```python
from build123d import *

# Parameters (mm, degrees)
F1_DEPTH = 9
F2_R     = 1.25
F3_DEPTH = 1
F4_R     = 0.625
F5_R     = 0.625
F6_DEPTH = 1


with BuildPart() as f1:
    # F0 (on Top) → F1 (new body)
    with BuildSketch(Plane.XY):
        with BuildLine():
            Line((-24.9881935865, -2), (-29.9881935865, -2))
            add(Edge.make_bspline(
                [(-29.9881935865, -2), (-30.1957792579, -1.9806863621), (-30.8858297438, -1.9886899929), (-30.9737131442, -1.9691203625), (-32.3240056363, -2.0563246792), (-32.4695344233, -2.4918309621)],
                knots=[0, 0, 0, 0, 0.3435850183, 0.5315375028, 0.9674384772, 0.9674384772, 0.9674384772, 0.9674384772], degree=3))
            Line((-32.4695344233, -2.4918309621), (-32.4881935865, -10.0656754612))
            ThreePointArc((-32.4881935865, -10.0656754612), (-31.3797872361, -10.9135774988), (-29.9881935865, -11.0183134402))
            Line((-29.9881935865, -11.0183134402), (-25.0104854877, -11.0483904604))
            ThreePointArc((-25.0104854877, -11.0483904604), (-23.5833955913, -10.9234349089), (-22.4881935865, -10))
            Line((-22.4881935865, -10), (-22.4881935865, -2.6204695865))
            ThreePointArc((-22.4881935865, -2.6204695865), (-23.6846353493, -2.0944376038), (-24.9881935865, -2))
        make_face()
        Polygon((-27.4881935865, 0), (-29.9881935865, 0), (-29.9881935865, -2), (-24.9881935865, -2), (-24.9881935865, 0), align=None)
        Polygon((-25.0104854877, -11.0483904604), (-29.9881935865, -11.0183134402), (-29.9881935865, -12), (-27.4881935865, -12), (-25.0128299031, -12), align=None)
    extrude(amount=F1_DEPTH)

    # F2 (on face) → F3 (join)
    with BuildSketch(Plane.XY.offset(9)):
        with Locations((-29.9974028021, -3.6542222369)):
            Circle(F2_R)
        with Locations((-24.9764043838, -3.7198562641)):
            Circle(F2_R)
        with BuildLine():
            Line((-24.4942996651, -8.7319174781), (-30.507825315, -8.6252950132))
            ThreePointArc((-30.507825315, -8.6252950132), (-27.5242896541, -9.9886223537), (-24.4942996651, -8.7319174781))
        make_face()
    extrude(amount=F3_DEPTH)

    # F4 (on face) + F5 (on face) → F6 (cut)
    with BuildSketch(Plane.XY.offset(10)):
        with Locations((-29.9974028021, -3.6542222369)):
            Circle(F4_R)
    with BuildSketch(Plane.XY.offset(10)):
        with Locations((-24.9764043838, -3.7198562641)):
            Circle(F5_R)
    extrude(amount=F6_DEPTH, mode=Mode.SUBTRACT)


solid = f1.part
```
CAD build for the part. Positions are in the model's coordinates, mm. A direction names the side the tool comes from. Round coordinates to 2 decimals unless told otherwise and drop trailing zeros. Order: outer loops, then holes, each group sorted by start corner. A loop starts at its lowest first (then second) coordinate and runs counter-clockwise, first axis right, second up.
Item 1: Tool access for faces 4 (the face through (-28, -6, 0)), 5 (the face through (-31.246, -3.599, 9.493)): list every direction of +Z, -Z, +X, -X, +Y, -Y with a clear straight run to the whole face (end or side of a thin tool).
Item 2: Saw through at B-B on y = -3. Write the cut outline in (x, z), then the cut area to 3 significant figures.
Item 3: Saw through at C-C on x = -28.5. Write the cut outline in (y, z).
Item 4: Saw through at A-A on x = -25.75. Write the cut outline in (y, z), then the cut area to 3 significant figures.
Item 5: Probe line 1 along Z through (x, y) = (-25.25, -8); line 2 along X through (y, z) = (-9, 6.5); line 3 along X through (y, z) = (-10.5, 7). List the from-to ranges inside material, lowest first.
Item 6: Mould opens along X. For faces 1 (the face through (-31.398, -10.906, 4.437)), 2 (the face through (-28, -9, 10)), 3 (the face through (-22.488, -6, 4)) say: pulls with the +X half, pulls with the -X half, needs draft (parallel to the pull), parting line crosses it, or undercut.
Item 7: Saw through at D-D on y = -8. Write the cut outline in (x, z), then the cut area to 3 significant figures.
Item 8: Pin check, flat tips, straight feed: pin 1 (3 mm diameter, centred on y = -2, z = 1, fed in from -X); pin 2 (1.6 mm diameter, centred on y = -1.5, z = 6.5, fed in from +X). Stop position of each tip, or through.
Reported:
1. face 4: -Z, +X, -X, +Y, -Y
1. face 5: +Z
2. outline: (-32.47, 0) - (-22.49, 0) - (-22.49, 9) - (-23.95, 9) - (-23.95, 10) - (-26, 10) - (-26, 9) - (-28.93, 9) - (-28.93, 10) - (-31.06, 10) - (-31.06, 9) - (-32.47, 9) - close
2. area: 94.0 mm2
3. outline: (-12, 0) - (0, 0) - (0, 9) - (-8.66, 9) - (-8.66, 10) - (-9.85, 10) - (-9.85, 9) - (-12, 9) - close
4. outline: (-12, 0) - (0, 0) - (0, 9) - (-2.74, 9) - (-2.74, 10) - (-4.7, 10) - (-4.7, 9) - (-8.71, 9) - (-8.71, 10) - (-9.62, 10) - (-9.62, 9) - (-12, 9) - close
4. area: 111 mm2
5. line 1: z = 0 to 9
5. line 2: x = -32.49 to -22.49
5. line 3: x = -32.08 to -22.91
6. face 1: undercut
6. face 2: needs draft
6. face 3: pulls with the +X half
7. outline: (-32.48, 0) - (-22.49, 0) - (-22.49, 9) - (-32.48, 9) - close
7. area: 90.0 mm2
8. pin 1: stops at x = -32.47
8. pin 2: stops at x = -23.08
